Autodesk Inventor part; units mm, degrees
ref_plane "YZ Plane" through (0, 0, 0) normal (1, 0, 0) x (0, 1, 0)
ref_plane "XZ Plane" through (0, 0, 0) normal (0, 1, 0) x (-1, 0, 0)
ref_plane "XY Plane" through (0, 0, 0) normal (0, 0, 1) x (1, 0, 0)
sketch "Sketch1" plane through (0, 0, 0) normal (0, 1, 0) x (-1, 0, 0)
  line L0 (0, 0) -> (22, 0)
  line L1 (22, 0) -> (22, -34)
  line L2 (22, -34) -> (0, -34)
  line L3 (0, -34) -> (0, 0)
  dimension "d0" = 22
  dimension "d1" = 34
extrude "Extrusion1" add sketch "Sketch1" along normal blind 4
sketch "Sketch2" plane through (0, 4, 0) normal (0, 1, 0) x (1, 0, 0)
  line L0 (-22, 0) -> (0, 0)
  circle A0 centre (-5, 5) radius 2.125
  dimension "d7" = 4.25
extrude "Extrusion2" cut sketch "Sketch2" against normal through all
pattern_linear "Rectangular Pattern1" count 3 spacing 6 along (-1, 0, 0) count 2 spacing 24 along (0, 0, -1) of "Extrusion2"
sketch "Sketch3" plane through (-22, 0, -34) normal (-1, 0, 0) x (0, 0, 1)
  line L0 (34, 0) -> (0, 0)
  line L1 (0, 0) -> (0, 4)
  line L2 (0, 4) -> (34, 4)
  line L3 (34, 4) -> (34, 0)
extrude "Extrusion3" add sketch "Sketch3" along normal blind 23.25
sketch "Sketch4" plane through (0, 4, 0) normal (0, 1, 0) x (1, 0, 0)
  line L0 (-45.25, 0) -> (-50.75, 0)
  line L1 (-50.75, 0) -> (-50.75, 34)
  line L2 (-50.75, 34) -> (-45.25, 34)
  line L3 (-45.25, 34) -> (-45.25, 0)
  point P0 (0, 0)
  dimension "d18" = 5.5
extrude "Extrusion4" add sketch "Sketch4" against normal blind 16.5
sketch "Sketch5" plane through (-50.75, 4, -34) normal (-1, 0, 0) x (0, 0, 1)
  line L0 (0, -4) -> (0, -16.5)
  line L1 (34, -16.5) -> (0, -16.5)
  line L2 (0, -16.5) -> (0, -10.25)
  line L3 (0, -10.25) -> (34, -10.25)
  line L4 (34, -10.25) -> (34, -16.5)
  point P0 (34, -4)
  dimension "d21" = 6.25
extrude "Extrusion5" add sketch "Sketch5" along normal blind 2
sketch "Sketch6" plane through (0, 0, -34) normal (0, 0, -1) x (-1, 0, 0)
  line L0 (52.75, -6.25) -> (45.25, -6.25)
  line L1 (45.25, -6.25) -> (45.25, -12.5)
  line L2 (45.25, -12.5) -> (52.75, -12.5)
  line L3 (52.75, -12.5) -> (52.75, -6.25)
  point P0 (0, 0)
extrude "Extrusion6" add sketch "Sketch6" along normal blind 6
sketch "Sketch7" plane through (0, 0, 0) normal (0, 0, 1) x (1, 0, 0)
  line L0 (-52.75, -12.5) -> (-45.25, -12.5)
  line L1 (-45.25, -12.5) -> (-45.25, -6.25)
  line L2 (-45.25, -6.25) -> (-52.75, -6.25)
  line L3 (-52.75, -6.25) -> (-52.75, -12.5)
  point P0 (0, 0)
extrude "Extrusion7" add sketch "Sketch7" along normal blind 6
fillet "Fillet1" radius 3 1 edges at (-52.75, -9.375, 6)
fillet "Fillet2" radius 3 1 edges at (-45.25, -9.375, 6)
fillet "Fillet3" radius 3 1 edges at (-52.75, -9.375, -40)
fillet "Fillet4" radius 3 1 edges at (-45.25, -9.375, -40)
sketch "Sketch8" plane through (0, -12.5, 0) normal (0, -1, 0) x (1, 0, 0)
  line L0 (-45.25, -34) -> (-52.75, -34)
  line L1 (-52.75, 3) -> (-52.75, -37)
  line L2 (-45.25, -34) -> (0, -34)
  line L3 (-49.75, -40) -> (-48.25, -40)
  line L4 (-49, -40) -> (-49, -34)
  line L5 (-45.25, -34) -> (-50.75, -34)
  line L6 (-52.75, 0) -> (-45.25, 0)
  line L7 (-50.75, 0) -> (-45.25, 0)
  line L8 (-49.75, 6) -> (-48.25, 6)
  line L9 (-49, 6) -> (-49, 0)
  circle A0 centre (-49, -37) radius 1.5
  circle A1 centre (-49, 3) radius 1.5
  point P0 (0, 0)
  dimension "d32" = 3
  dimension "d33" = 3
extrude "Extrusion8" cut sketch "Sketch8" against normal through all
sketch "Sketch9" plane through (0, 4, 0) normal (0, 1, 0) x (1, 0, 0)
  line L0 (0, 0) -> (0, 34)
  line L1 (0, 17) -> (-24, 17)
  line L2 (-21.5, 12) -> (-26.5, 12)
  line L3 (-26.5, 12) -> (-26.5, 22)
  line L4 (-26.5, 22) -> (-21.5, 22)
  line L5 (-21.5, 22) -> (-21.5, 12)
  line L6 (-21.5, 12) -> (-26.5, 22) construction
  line L7 (-26.5, 12) -> (-21.5, 22) construction
  dimension "d36" = 24
  dimension "d37" = 5
  dimension "d38" = 10
extrude "Extrusion9" cut sketch "Sketch9" against normal through all
sketch "Sketch10" plane through (0, 0, 0) normal (1, 0, 0) x (0, 0, -1)
  line L0 (0, 4) -> (34, 4)
  line L1 (34, 4) -> (34, 0)
  line L2 (34, 0) -> (0, 0)
  line L3 (0, 0) -> (0, 4)
extrude "Extrusion10" add sketch "Sketch10" along normal blind 30
sketch "Sketch11" plane through (-45.25, -6.25, -34) normal (0, 0, -1) x (-1, 0, 0)
  line L0 (-75.25, 10.25) -> (-45.25, 10.25)
  line L1 (-45.25, 10.25) -> (-45.25, 6.25)
  line L2 (-45.25, 6.25) -> (-75.25, 6.25)
  line L3 (-75.25, 6.25) -> (-75.25, 10.25)
extrude "Extrusion11" add sketch "Sketch11" along normal blind 40
properties part number "CartServoMountV2"
Build history of the part. All positions in model axes, mm. A direction names the side the tool comes from. Give positions to 0.01 mm unless a question says otherwise; leave off trailing zeros. Loops run counter-clockwise (first coordinate to the right, second up) from the corner with the lowest first, then second, coordinate; pieces in that order, holes last. Notation, with made-up numbers: (33, 84.25) - (61, 84.25) arc R8 cw to (61, 98.25) - close; hole circle Ø4 at (29, 41). An arc over 180 degrees is marked (long way). Write item = value, one per line. Start each with the question number.
1) Tool access for faces 1 (the flat face through (-50.75, -1, -17)), 2 (the flat face through (-24, 2, -12)), 3 (the flat face through (-20, 1, 0)): list every direction of +Z, -Z, +X, -X, +Y, -Y with a clear straight run to the whole face (end or side of a thin tool).
2) Pull direction X, two halves, no side cores. Call faces 4 (the flat face through (-26, 1, -34)), 5 (the flat face through (-24, 2, -22)), 6 (the flat face through (-45.25, -6, -17)): +X half, -X half, draft (parallel to the pull), parting line (faces both ways), or undercut.
3) Band-saw the part on A-A on z = -15.5. Give the cut face in (x, y), plus the area to 3 significant figures.
4) Band-saw the part on B-B on z = -5. Give the cut face in (x, y) (3 decimals), plus the area to 3 significant figures.
5) Drop flat-ended pins along their axis: pin 1 Ø3 at (x, y) = (-23.5, 2) entering from +Z; pin 2 Ø1.2 at (y, z) = (2.5, -46) entering from -X; pin 3 Ø2 at (y, z) = (-4, -8.5) entering from -X. Give the stop position or say it passes through.
6) Band-saw the part on D-D on x = -17. Give the cut face in (y, z) (3 decimals).
7) Band-saw the part on C-C on y = -8. Give the cut face in (x, z).
8) Probe probe 1 along X at (y, z) = (2.5, -29) (3 decimals); probe 2 along Z at (x, y) = (-5, 1.25) (3 decimals); probe 3 along X at (y, z) = (-10, -37). List the from-to ranges inside material, lowest first. Write a range as from..to.
Final values:
q1.face_1 = +Z, -Z, -X, +Y
q1.face_2 = +Y, -Y
q1.face_3 = +Z, +X, -X, +Y
q2.face_4 = draft
q2.face_5 = undercut
q2.face_6 = +X half
q3.outline = (-52.75, -12.5) - (-45.25, -12.5) - (-45.25, 0) - (-26.5, 0) - (-26.5, 4) - (-50.75, 4) - (-50.75, -6.25) - (-52.75, -6.25) - close; (-21.5, 0) - (30, 0) - (30, 4) - (-21.5, 4) - close
q3.area = 384 mm²
q4.outline = (-52.75, -12.5) - (-45.25, -12.5) - (-45.25, 0) - (-19.125, 0) - (-19.125, 4) - (-50.75, 4) - (-50.75, -6.25) - (-52.75, -6.25) - close; (-14.875, 0) - (-13.125, 0) - (-13.125, 4) - (-14.875, 4) - close; (-8.875, 0) - (-7.125, 0) - (-7.125, 4) - (-8.875, 4) - close; (-2.875, 0) - (30, 0) - (30, 4) - (-2.875, 4) - close
q4.area = 353 mm²
q5.pin_1 = 0
q5.pin_2 = 0
q5.pin_3 = -50.75
q6.outline = (0, -34) - (4, -34) - (4, -31.125) - (0, -31.125) - close; (0, -26.875) - (4, -26.875) - (4, -7.125) - (0, -7.125) - close; (0, -2.875) - (4, -2.875) - (4, 0) - (0, 0) - close
q7.outline = (-52.75, -37) arc R3 ccw to (-49.75, -40) - (-48.25, -40) arc R3 ccw to (-45.25, -37) - (-45.25, 3) arc R3 ccw to (-48.25, 6) - (-49.75, 6) arc R3 ccw to (-52.75, 3) - close; hole circle Ø3 at (-49, -37); hole circle Ø3 at (-49, 3)
q8.probe_1 = -50.75..-19.125, -14.875..-13.125, -8.875..-7.125, -2.875..30
q8.probe_2 = -34..-31.125, -26.875..-7.125, -2.875..0
q8.probe_3 = -52.75..-50.5, -47.5..-45.25
